from build123d import *

# Parameters (mm, degrees)
EXTRUDE_1_DEPTH     = 30
FILLET_1_R          = 15
SKETCH_2_R          = 7
CUT_EXTRUDE_1_DEPTH = 82.853527719
EXTRUDE_START       = -11.5
EXTRUDE_3_DEPTH     = 7
CHAMFER_1_SIZE      = 9


with BuildPart() as part:
    # 스케치1 → 보스-돌출1 (new body)
    with BuildSketch(Plane.XY):
        Polygon((0, 0), (-70, 0), (-70, 30), (-41, 30), (-41, 9), (0, 9), align=None)
    extrude(amount=EXTRUDE_1_DEPTH)

    # 필렛1
    fillet_1_edges = [part.edges().sort_by_distance(p)[0] for p in [
        (-70, 15, 0),
        (-70, 15, 30),
    ]]
    fillet(fillet_1_edges, radius=FILLET_1_R - 0.0001)  # a hair under: the kernel refuses the full size

    # 스케치2 → 컷-돌출1 (cut, through all)
    with BuildSketch(Plane(origin=(0, 30, 0), x_dir=(1, 0, 0), z_dir=(0, 1, 0))):
        with Locations(Location((-55, -15, 0), (0, 0, 270))):
            Circle(SKETCH_2_R)
    extrude(amount=-CUT_EXTRUDE_1_DEPTH, mode=Mode.SUBTRACT)

    # 스케치3 → 보스-돌출3 (add)
    with BuildSketch(Plane.XY.offset(30).offset(EXTRUDE_START)):
        Polygon((0, 9), (-41, 30), (-41, 9), align=None)
    extrude(amount=-EXTRUDE_3_DEPTH)

    # 모따기1
    chamfer_1_edges = [part.edges().sort_by_distance(p)[0] for p in [
        (0, 4.5, 30),
        (0, 4.5, 0),
    ]]
    chamfer(chamfer_1_edges, length=CHAMFER_1_SIZE)


solid = part.part
Design review of the part built by this model. Coordinates are the model's own, in mm. A direction names the side the tool comes from. Coordinates: 2 decimals unless noted, no trailing zeros. Order: outer loops, then holes, each group sorted by start corner. A loop starts at its lowest first (then second) coordinate and runs counter-clockwise, first axis right, second up.
Item 1: Take a section at D-D, the plane x = -5.5. Write out the cut boundary in (y, z), then the cut area to 3 significant figures.
Item 2: For line 1 (Z direction, x = -38, y = 12); line 2 (Z direction, x = -49, y = 14.5); line 3 (Z direction, x = -50, y = 14.25), list the stretches that pass through material, from the lowest coordinate up.
Item 3: For faces 1 (the flat face through (-52, 30, 8)), 2 (the flat face through (-30, 15, 18.5)), 3 (the flat face through (-41, 20, 6)), list the 3-axis set-ups (+Z, -Z, +X, -X, +Y, -Y) from which the entire face can be reached by the end or side of a thin tool; tool diameter is ignored.
Item 4: For pin 1 Ø3.5 at (x, z) = (-24, 26) entering from +Y; pin 2 Ø10 at (x, z) = (-51.5, 6.5) entering from -Y; pin 3 Ø6.5 at (x, y) = (-17.5, 22.5) entering from +Z; pin 4 Ø3.5 at (y, z) = (15, 22) entering from +X, all flat-tipped, find the tip position at first contact; note any pin that passes through.
Item 5: The part is to be moulded in two halves that separate along X. For faces 4 (the flat face through (-36.8, 8.5, 0)), 5 (the cylindrical face through (-65.72, 15.21, 4.51)), 6 (the cylindrical face through (-48.06, 15.21, 14.09)), 7 (the flat face through (0, 5, 15)), say which applies: pulls with the +X half, pulls with the -X half, needs draft (parallel to the pull), parting line crosses it, or undercut.
Item 6: Take a section at B-B, the plane x = -27. Write out the cut boundary in (y, z).
The answers:
1. outline: (0, 3.5) - (9, 3.5) - (9, 11.5) - (11.82, 11.5) - (11.82, 18.5) - (9, 18.5) - (9, 26.5) - (0, 26.5) - close
1. area: 227 mm2
2. line 1: z = 11.5 to 18.5
2. line 2: z = 0 to 11.39, 18.61 to 30
2. line 3: z = 0 to 10.1, 19.9 to 30
3. face 1: +Z, -Z, +X, -X, +Y
3. face 2: +Z, +X, +Y
3. face 3: -Z, +X, +Y
4. pin 1: stops at y = 9
4. pin 2: stops at y = 0
4. pin 3: passes through
4. pin 4: stops at x = -41
5. face 4: needs draft
5. face 5: pulls with the -X half
5. face 6: undercut
5. face 7: pulls with the +X half
6. outline: (0, 0) - (9, 0) - (9, 11.5) - (22.83, 11.5) - (22.83, 18.5) - (9, 18.5) - (9, 30) - (0, 30) - close
